Input: part model. Units: mm. Frame: model coordinates. A direction names the side the tool comes from. Round coordinates to 2 decimals unless told otherwise and drop trailing zeros. Write each loop counter-clockwise with the first axis right and the second up, starting at its lowest first coordinate (ties: lowest second). Pieces come first, ordered by that corner, then holes. Notation, with made-up numbers: M -32,79.25 L -28,79.25 A35 ccw -28,118.25 Z; hole C 78.5,75 d8. An arc over 180 degrees is marked long. Use one line per item in the form item = value. Start each with the question number.
```python
from build123d import *

# Parameters (mm, degrees)
SKETCH052_R       = 13
SKETCH052_R_2     = 6
SKETCH052_R_3     = 4
PAD027_DEPTH      = 8
PAD028_DEPTH      = 35
CYLINDER016_R     = 3.75
CYLINDER016_DEPTH = 40
CYLINDER017_R     = 3.75
CYLINDER017_DEPTH = 30
CYLINDER018_R     = 2.5
CYLINDER018_DEPTH = 50
CYLINDER019_R     = 2.5
CYLINDER019_DEPTH = 40
CYLINDER020_R     = 2.5
CYLINDER020_DEPTH = 40
FILLET022_R       = 3.5
FILLET023_R       = 2


with BuildPart() as part:
    # Sketch052 → Pad027 (new body)
    with BuildSketch(Plane.XY):
        with BuildLine():
            Line((0, 0), (0, 60))
            Line((0, 60), (110, 60))
            Line((110, 60), (110, 40))
            ThreePointArc((110, 40), (60.755711, 29.54965), (20, 0))
            Line((20, 0), (0, 0))
        make_face()
        with Locations((25, 35)):
            Circle(SKETCH052_R, mode=Mode.SUBTRACT)
        with Locations((58, 43)):
            Circle(SKETCH052_R_2, mode=Mode.SUBTRACT)
        with Locations((85, 45)):
            Circle(SKETCH052_R_3, mode=Mode.SUBTRACT)
    extrude(amount=PAD027_DEPTH)

    # Sketch053 (on Face10 of Pad027) → Pad028 (join)
    with BuildSketch(Plane.XY.offset(8)):
        Polygon((0, 0), (0, 60), (110, 60), (110, 53), (7, 53), (7, 0), align=None)
    extrude(amount=PAD028_DEPTH)

    # Cylinder016 → Cylinder016 (cut)
    with BuildSketch(Plane(origin=(0, 45, 25), x_dir=(0, 1, 0), z_dir=(1, 0, 0))):
        Circle(CYLINDER016_R)
    extrude(amount=CYLINDER016_DEPTH, mode=Mode.SUBTRACT)

    # Cylinder017 → Cylinder017 (cut)
    with BuildSketch(Plane(origin=(0, 16, 25), x_dir=(0, 1, 0), z_dir=(1, 0, 0))):
        Circle(CYLINDER017_R)
    extrude(amount=CYLINDER017_DEPTH, mode=Mode.SUBTRACT)

    # Cylinder018 → Cylinder018 (cut)
    with BuildSketch(Plane(origin=(30, 70, 25), x_dir=(1, 0, 0), z_dir=(0, -1, 0))):
        Circle(CYLINDER018_R)
    extrude(amount=CYLINDER018_DEPTH, mode=Mode.SUBTRACT)

    # Cylinder019 → Cylinder019 (cut)
    with BuildSketch(Plane(origin=(60, 70, 25), x_dir=(1, 0, 0), z_dir=(0, -1, 0))):
        Circle(CYLINDER019_R)
    extrude(amount=CYLINDER019_DEPTH, mode=Mode.SUBTRACT)

    # Cylinder020 → Cylinder020 (cut)
    with BuildSketch(Plane(origin=(90, 70, 25), x_dir=(1, 0, 0), z_dir=(0, -1, 0))):
        Circle(CYLINDER020_R)
    extrude(amount=CYLINDER020_DEPTH, mode=Mode.SUBTRACT)

    # Fillet022
    fillet022_edges = [part.edges().sort_by_distance(p)[0] for p in [
        (0, 60, 25.5),
        (7, 53, 25.5),
        (0, 0, 25.5),
        (7, 26.5, 8),
        (58.5, 53, 8),
        (110, 40, 4),
        (110, 60, 25.5),
    ]]
    fillet(fillet022_edges, radius=FILLET022_R)

    # Fillet023
    fillet023_edges = [part.edges().sort_by_distance(p)[0] for p in [
        (59.206101, 28.847876, 8),
        (15.25, 0, 8),
        (7, 24.75, 43),
        (55, 60, 43),
    ]]
    fillet(fillet023_edges, radius=FILLET023_R)


solid = part.part
```
Item 1: Cut plane A-A (z = 25). Give the number of separate pieces and of enclosed holes in the cut face, plus the area to 3 significant figures.
Item 2: Cut plane B-B (z = 20). Output: boundary loops of the cut face in (x, y), plus the area to 3 significant figures.
Item 3: Reachability of faces 1 (the face through (109.43, 53.6, 26.04)), 2 (the face through (0, 30, 20)) from +Z, -Z, +X, -X, +Y, -Y: full face, straight path, thin tool, end or side. Return the list, or none.
Item 4: First-contact query: pin 1 (4.5 mm diameter, centred on y = 45, z = 25, fed in from +X); pin 2 (6 mm diameter, centred on y = 45.5, z = 7.5, fed in from +X); pin 3 (12 mm diameter, centred on y = 32, z = 22.5, fed in from +X); pin 4 (10 mm diameter, centred on x = 36.5, y = 41, fed in from +Z). Flat tips, straight axial feed; report the tip coordinate or a pass-through.
Item 5: Draft query along Y for faces 3 (the face through (49, 35, 8)), 4 (the face through (15.18, 0.57, 7.4)), 5 (the face through (88.695, 43.468, 3.944)). Return one class per face: +Y half, -Y half, draft (parallel to the pull), parting line (faces both ways), or undercut.
Item 6: Ray query, line 1 (Y direction, x = 3, z = 25); line 2 (Z direction, x = 60, y = 55.5); line 3 (X direction, y = 20, z = 34.5). Return the intervals inside material, ascending. Write a range as from..to.
Final values:
q1.separate_pieces = 6
q1.enclosed_holes = 0
q1.area = 924 mm^2
q2.outline = M 0,3.5 A3.5 ccw 3.5,0 L 5,0 A2 ccw 7,2 L 7,49.5 A3.5 cw 10.5,53 L 108,53 A2 ccw 110,55 L 110,56.5 A3.5 ccw 106.5,60 L 3.5,60 A3.5 ccw 0,56.5 Z
q2.area = 1,130 mm^2
q3.face_1 = +Z, +X, -Y
q3.face_2 = +Z, -Z, -X, +Y, -Y
q4.pin_1 = through
q4.pin_2 = 110
q4.pin_3 = 7
q4.pin_4 = 8
q5.face_3 = draft
q5.face_4 = -Y half
q5.face_5 = undercut
q6.line_1 = 0.04..12.25, 19.75..41.25, 48.75..59.96
q6.line_2 = 0..22.5, 27.5..43
q6.line_3 = 0..7
